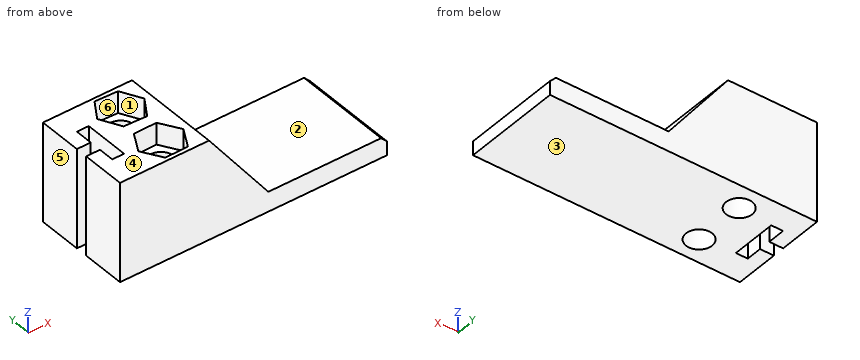
from build123d import *

# Parameters (mm, degrees)
F1_DEPTH       = 25
F2_DEPTH       = 25
F4_D           = 13.2
F4_CBORE_D     = 23
F4_CBORE_DEPTH = 0
F6_DEPTH       = 50.001
F8_DEPTH       = 11
F9_SIZE        = 3


# Not quite as in the source:
# - a feature names something its author has since deleted; it is built from what else it names


with BuildPart() as f1:
    # F0 (on Front) → F1 (new body, symmetric)
    with BuildSketch(Plane.XZ):
        Polygon((67.5, -5), (67.5, 5), (7.5, 5), (-67.5, 5), (-67.5, -5), align=None)
    extrude(amount=F1_DEPTH, both=True)

    # F0 (on Front) → F2 (join, symmetric)
    with BuildSketch(Plane.XZ):
        Polygon((-67.5, 5), (7.5, 5), (-22.5, 45), (-67.5, 45), align=None)
    extrude(amount=F2_DEPTH, both=True)

    # F4 (through all)
    with Locations(Plane(origin=(0, 0, -5), x_dir=(1, 0, 0), z_dir=(0, 0, -1))):
        with Locations((-37.5, 13), (-37.5, -13)):
            CounterBoreHole(F4_D / 2, F4_CBORE_D / 2, F4_CBORE_DEPTH)

    # F5 (on face) → F6 (cut, through all)
    with BuildSketch(Plane.XY.offset(45)):
        Polygon((-60.5, 3), (-67.5, 3), (-67.5, -3), (-60.5, -3), (-60.5, -10.9647801146), (-54.5, -10.9647801146), (-54.5, 11.965367943), (-60.5, 11.965367943), align=None)
    extrude(amount=-F6_DEPTH, mode=Mode.SUBTRACT)

    # F7 (on face) → F8 (cut)
    with BuildSketch(Plane.XY.offset(45)):
        Polygon((-25.954678559, -12.8028042668), (-31.898115794, -2.9028604706), (-43.443437235, -3.1000562039), (-49.045321441, -13.1971957332), (-43.101884206, -23.0971395294), (-31.556562765, -22.8999437961), align=None)
        Polygon((-25.9640170016, 12.4955898546), (-31.2951765009, 22.7382492615), (-42.8311594993, 23.2426594069), (-49.0359829984, 13.5044101454), (-43.7048234991, 3.2617507385), (-32.1688405007, 2.7573405931), align=None)
    extrude(amount=-F8_DEPTH, mode=Mode.SUBTRACT)

    # F9
    f9_edges = [f1.edges().sort_by_distance(p)[0] for p in [
        (67.5, 0, 5),
    ]]
    chamfer(f9_edges, length=F9_SIZE)


solid = f1.part
Model file for the job. Use its own axes, mm. Face numbers are marked on the shaded views. A direction names the side the tool comes from. Round coordinates to 2 decimals unless told otherwise and drop trailing zeros. Loops run counter-clockwise (first coordinate to the right, second up) from the corner with the lowest first, then second, coordinate; pieces in that order, holes last. Notation, with made-up numbers: (42, 61.5) -> (95, 61.5) arc R14 cw to (95, 87.5) -> close; hole circle Ø2 at (-22, 75.25). An arc over 180 degrees is marked (long way). Answer as CSV lines item,"result". Start each with the question number.
1) Mould opens along X. For the marked faces 4, 5 and 6 say: +X half, -X half, draft (parallel to the pull), parting line (faces both ways), or undercut.
2) Pin check, flat tips, straight feed: P1, Ø10, axis at x = -39.5, y = -13.5, coming from the +Z side; P2, Ø2.5, axis at y = -5, z = 27, coming from the +X side; P3, Ø5, axis at y = -5, z = 35.5, coming from the +X side. Stop position of each tip, or through.
3) Probe line 1 along Y through (x, z) = (-38, 28); line 2 along Y through (x, z) = (-35, 26.5); line 3 along X through (y, z) = (-3.5, 1). List the from-to ranges inside material, lowest first.
4) Slice it at B-B (x = -37.5). List the corners of the cut face in (y, z).
5) Slice it at A-A (z = 41). List the corners of the cut face in (x, y).
6) Tool access for the marked faces 1, 2 and 3: list every direction of +Z, -Z, +X, -X, +Y, -Y with a clear straight run to the whole face (end or side of a thin tool).
7) Slice it at C-C (x = 9). List the corners of the cut face in (y, z).
8) Slice it at D-D (z = 31.5). List the corners of the cut face in (x, y) (3 decimals).
Filled in:
1,face 4,"draft"
1,face 5,"-X half"
1,face 6,"undercut"
2,P1,"stops at z = 34"
2,P2,"stops at x = -8.06"
2,P3,"stops at x = -13.5"
3,line 1,"y = -25 to -19.58, -6.42 to 6.42, 19.58 to 25"
3,line 2,"y = -25 to -19.11, -6.89 to 6.89, 19.11 to 25"
3,line 3,"x = -67.5 to -60.5, -54.5 to 67.5"
4,outline,"(-25, -5) -> (-19.6, -5) -> (-19.6, 34) -> (-23, 34) -> (-23, 45) -> (-25, 45) -> close; (-6.4, -5) -> (6.4, -5) -> (6.4, 34) -> (2.99, 34) -> (2.99, 45) -> (-3, 45) -> (-3, 34) -> (-6.4, 34) -> close; (19.6, -5) -> (25, -5) -> (25, 45) -> (23.01, 45) -> (23.01, 34) -> (19.6, 34) -> close"
5,outline,"(-67.5, -25) -> (-19.5, -25) -> (-19.5, 25) -> (-67.5, 25) -> (-67.5, 3) -> (-60.5, 3) -> (-60.5, 11.97) -> (-54.5, 11.97) -> (-54.5, -10.96) -> (-60.5, -10.96) -> (-60.5, -3) -> (-67.5, -3) -> close; hole (-49.05, -13.2) -> (-43.1, -23.1) -> (-31.56, -22.9) -> (-25.95, -12.8) -> (-31.9, -2.9) -> (-43.44, -3.1) -> close; hole (-49.04, 13.5) -> (-43.7, 3.26) -> (-32.17, 2.76) -> (-25.96, 12.5) -> (-31.3, 22.74) -> (-42.83, 23.24) -> close"
6,face 1,"+Z"
6,face 2,"+Z, +X, +Y, -Y"
6,face 3,"-Z, +X, -X, +Y, -Y"
7,outline,"(-25, -5) -> (25, -5) -> (25, 5) -> (-25, 5) -> close"
8,outline,"(-67.5, -25) -> (-12.375, -25) -> (-12.375, 25) -> (-67.5, 25) -> (-67.5, 3) -> (-60.5, 3) -> (-60.5, 11.965) -> (-54.5, 11.965) -> (-54.5, -10.965) -> (-60.5, -10.965) -> (-60.5, -3) -> (-67.5, -3) -> close; hole circle Ø13.2 at (-37.5, -13); hole circle Ø13.2 at (-37.5, 13)"
